Work out the finished part from the listing and answer in its coordinate system (mm). Face numbers are marked on the shaded views. A direction names the side the tool comes from. Give positions to 0.01 mm unless a question says otherwise; leave off trailing zeros. Order: outer loops, then holes, each group sorted by start corner. A loop starts at its lowest first (then second) coordinate and runs counter-clockwise, first axis right, second up. Notation, with made-up numbers: (-21, -32) -> (-1, -32) arc R23 cw to (-1, -23) -> close; hole circle Ø8 at (5.25, -1). An arc over 180 degrees is marked (long way). Answer as CSV lines item,"result". Start each with the question number.
1. A cutting plane is placed at A-A (y = 4.5). Give the vertices of the cut face in (x, z), then the cut area to 3 significant figures.
2. Flat-ended cylindrical pins translate along their axes: pin 1 (15.5 mm diameter, centred on x = -0.5, y = 18.5, fed in from -Z); pin 2 (8 mm diameter, centred on x = 31.5, z = 10, fed in from -Y); pin 3 (3 mm diameter, centred on x = -41, z = 5.5, fed in from -Y); pin 4 (9.5 mm diameter, centred on y = 15.5, z = 14, fed in from +X). Find the tip coordinate at first contact, or state that the pin passes through.
3. A cutting plane is placed at C-C (x = -32.5). Give the vertices of the cut face in (y, z) (1 decimal), then the cut area to 3 significant figures.
4. For the marked faces 5, 6 and 7, determine the directions among +Z, -Z, +X, -X, +Y, -Y from which every point of the face is accessible in a straight line to the end or side of a thin tool.
5. Find the intervals of material crossed by L1, parallel to X at y = 6.5, z = 2.75; L2, parallel to Y at x = 36.5, z = 11.75; L3, parallel to X at y = 4, z = 7.75, in increasing order.
6. For a pull along Y with two mould halves and no side action, classify the marked faces 1, 2, 3 and 4 as released by +Y, released by -Y, zero draft, split by the parting line, or undercut.
7. A cutting plane is placed at B-B (z = 5.25). State how many separate pieces and enclosed holes the cut face has, then the cut area to 3 significant figures.
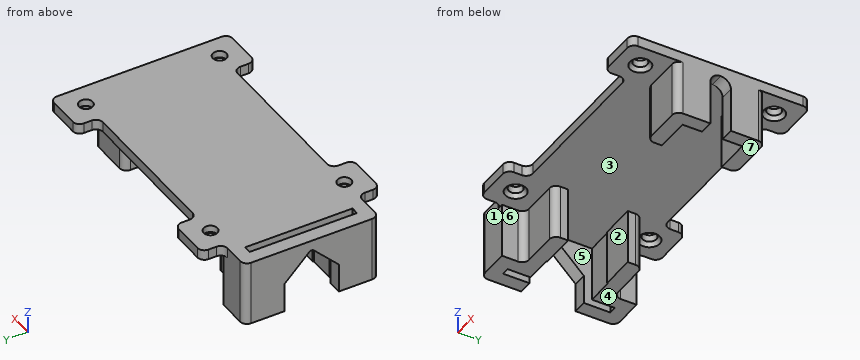
Autodesk Inventor part; units mm, degrees
ref_plane "YZ Plane" through (0, 0, 0) normal (1, 0, 0) x (0, 1, 0)
ref_plane "XZ Plane" through (0, 0, 0) normal (0, 1, 0) x (-1, 0, 0)
ref_plane "XY Plane" through (0, 0, 0) normal (0, 0, 1) x (1, 0, 0)
sketch "Sketch1" plane through (0, 0, 0) normal (0, 0, 1) x (1, 0, 0)
  line L0 (-33.557, 36.1315) -> (-43.657, 36.1315)
  line L1 (-43.657, 36.1315) -> (-43.657, -3.0685)
  line L2 (-43.657, -3.0685) -> (-33.457, -3.0685)
  line L3 (40.043, 3.5815) -> (40.043, 29.4815)
  line L4 (35.943, 25.1065) -> (35.943, 7.9565) construction
  line L5 (35.943, 7.9565) -> (-29.957, 7.9565) construction
  line L6 (35.943, 25.1065) -> (-29.957, 25.1065) construction
  line L7 (-37.557, 25.3815) -> (-29.957, 25.3815) construction
  line L8 (-29.957, 7.6815) -> (-29.957, 25.3815) construction
  line L9 (-37.557, 7.6815) -> (-29.957, 7.6815) construction
  line L10 (-37.557, 1.0315) -> (-37.557, 6.1295) construction
  line L11 (-39.557, 1.0315) -> (-37.557, 1.0315) construction
  line L12 (-39.557, 6.1295) -> (-39.557, 1.0315) construction
  line L13 (-39.557, 13.2232) -> (-39.557, 6.1295) construction
  line L14 (-39.557, 19.8398) -> (-39.557, 13.2232) construction
  line L15 (-39.557, 26.9336) -> (-39.557, 19.8398) construction
  line L16 (-39.557, 32.0315) -> (-39.557, 26.9336) construction
  line L17 (-39.557, 32.0315) -> (-37.557, 32.0315) construction
  line L18 (-37.557, 26.9336) -> (-37.557, 32.0315) construction
  line L19 (-37.557, 19.8398) -> (-37.557, 26.9336) construction
  line L20 (-37.557, 6.1295) -> (-37.557, 13.2232) construction
  line L21 (-33.557, 36.1315) -> (-33.557, 29.4815) construction
  line L22 (-33.557, 29.4815) -> (40.043, 29.4815) construction
  line L23 (35.943, 25.1065) -> (-29.957, 25.1065) construction
  line L24 (-29.957, 25.3815) -> (-29.957, 25.1065) construction
  line L25 (-29.957, 25.3815) -> (-37.557, 25.3815) construction
  line L26 (-37.557, 25.3815) -> (-37.557, 32.0315) construction
  line L27 (-37.557, 32.0315) -> (-39.557, 32.0315) construction
  line L28 (-39.557, 32.0315) -> (-39.557, 1.0315) construction
  line L29 (-39.557, 1.0315) -> (-37.557, 1.0315) construction
  line L30 (-37.557, 1.0315) -> (-37.557, 7.6815) construction
  line L31 (-37.557, 7.6815) -> (-29.957, 7.6815) construction
  line L32 (-29.957, 7.6815) -> (-29.957, 7.9565) construction
  line L33 (-29.957, 7.9565) -> (35.943, 7.9565) construction
  line L34 (35.943, 7.9565) -> (35.943, 25.1065) construction
  line L35 (-29.857, 7.8565) -> (36.043, 7.8565)
  line L36 (36.043, 7.8565) -> (36.043, 25.2065)
  line L37 (36.043, 25.2065) -> (-29.857, 25.2065)
  line L38 (-29.857, 25.2065) -> (-29.857, 25.4815)
  line L39 (-29.857, 25.4815) -> (-37.457, 25.4815)
  line L40 (-37.457, 25.4815) -> (-37.457, 32.1315)
  line L41 (-37.457, 32.1315) -> (-39.657, 32.1315)
  line L42 (-39.657, 32.1315) -> (-39.657, 0.9315)
  line L43 (-39.657, 0.9315) -> (-37.457, 0.9315)
  line L44 (-37.457, 0.9315) -> (-37.457, 7.5815)
  line L45 (-37.457, 7.5815) -> (-29.857, 7.5815)
  line L46 (-29.857, 7.5815) -> (-29.857, 7.8565)
  line L47 (-33.557, 36.1315) -> (-33.557, 29.4815)
  line L48 (-33.557, 29.4815) -> (40.043, 29.4815)
  line L49 (-33.457, -3.0685) -> (-33.457, 3.5815)
  line L50 (-33.457, 3.5815) -> (40.043, 3.5815)
  line L51 (-33.457, 36.1315) -> (-33.557, 36.1315)
  line L52 (-33.457, 36.1315) -> (-33.557, 36.1315)
  point P0 (0, 0)
  dimension "d6" = 0.1
  dimension "d7" = 4
  dimension "d8" = 4
  dimension "d9" = 4
  dimension "d10" = 4
  dimension "d11" = 4
  dimension "d12" = 4
  dimension "d13" = 4
  dimension "d14" = 4
extrude "Extrusion1" add sketch "Sketch1" along normal blind 16
sketch "Sketch2" plane through (0, 0, 16) normal (0, 0, 1) x (1, 0, 0)
  line L0 (-43.657, 36.1315) -> (-43.657, -3.0685)
  line L1 (-43.657, -3.0685) -> (-43.657, 36.1315)
  line L2 (40.043, 36.1315) -> (40.043, -3.0685)
  line L3 (-43.657, -3.0685) -> (-33.457, -3.0685)
  line L4 (40.043, 3.5815) -> (40.043, 29.4815)
  line L5 (40.043, 29.4815) -> (27.043, 29.4815) construction
  line L6 (27.043, 36.1315) -> (27.043, 42.4815)
  line L7 (27.043, 42.4815) -> (40.043, 42.4815)
  line L8 (40.043, 42.4815) -> (40.043, 29.4815)
  line L9 (-33.557, 29.4815) -> (-33.557, 36.1315) construction
  line L10 (-33.557, 29.4815) -> (-20.557, 29.4815) construction
  line L11 (-20.557, 36.1315) -> (-20.557, 42.4815)
  line L12 (-20.557, 42.4815) -> (-33.557, 42.4815)
  line L13 (-33.557, 42.4815) -> (-33.557, 36.1315)
  line L14 (-33.457, 3.5815) -> (40.043, 3.5815) construction
  line L15 (-20.557, 3.5815) -> (-20.457, 3.5815)
  line L16 (-20.457, -3.0685) -> (-20.457, -9.4185)
  line L17 (-20.457, -9.4185) -> (-33.457, -9.4185)
  line L18 (-33.457, -9.4185) -> (-33.457, -3.0685)
  line L19 (40.043, 3.5815) -> (27.043, 3.5815) construction
  line L20 (27.043, -3.0685) -> (27.043, -9.4185)
  line L21 (27.043, -9.4185) -> (40.043, -9.4185)
  line L22 (40.043, -9.4185) -> (40.043, 3.5815)
  line L23 (27.043, -3.0685) -> (-20.457, -3.0685)
  line L24 (-33.457, -3.0685) -> (-43.657, -3.0685)
  line L25 (-43.657, 36.1315) -> (-33.557, 36.1315)
  line L26 (-20.557, 36.1315) -> (27.043, 36.1315)
  point P0 (0, 0)
  point P1 (-38.557, -3.0685)
  point P2 (40.043, 16.5315)
  dimension "d60" = 13
  dimension "d61" = 13
  dimension "d62" = 13
  dimension "d63" = 13
  dimension "d64" = 13
  dimension "d65" = 13
  dimension "d66" = 13
  dimension "d67" = 13
extrude "Extrusion2" add sketch "Sketch2" along normal blind 3
sketch "Sketch3" plane through (40.043, 3.5815, 0) normal (1, 0, 0) x (0, 0, -1)
  line L0 (0, 15.95) -> (-16, 15.95)
  line L1 (-16, 15.95) -> (-16, 9.95)
  line L2 (-16, 9.95) -> (0, 9.95)
  line L3 (0, 9.95) -> (0, 15.95)
  line L4 (0, 0) -> (0, 25.9) construction
  line L5 (0, 25.9) -> (-16, 25.9) construction
  line L6 (0, 0) -> (-16, 0) construction
  line L7 (-16, 21.625) -> (-16, 4.275) construction
  point P0 (0, -3.5815)
  point P1 (0, 12.95)
  dimension "d19" = 6
  dimension "d21" = 0
extrude "Extrusion3" cut sketch "Sketch3" against normal blind 4
fillet "Fillet1" radius 3 2 edges at (38.043, 19.5315, 16) (38.043, 13.5315, 16)
sketch "Sketch4" plane through (-43.657, -3.0685, 0) normal (-1, 0, 0) x (0, 0, 1)
  line L0 (0, 27.5) -> (16, 27.5)
  line L1 (16, 27.5) -> (16, 11.7)
  line L2 (16, 11.7) -> (0, 11.7)
  line L3 (0, 11.7) -> (0, 27.5)
  line L4 (0, 39.2) -> (0, 0) construction
  line L5 (0, 39.2) -> (19, 39.2) construction
  line L6 (0, 0) -> (19, 0) construction
  line L7 (19, 39.2) -> (19, 0) construction
  point P0 (0, 3.0685)
  point P1 (0, 19.6)
  dimension "d25" = 15.8
  dimension "d28" = 11.7
  dimension "d29" = 11.7
  dimension "d30" = 3
extrude "Extrusion4" cut sketch "Sketch4" against normal blind 4
chamfer "Chamfer1" distance 7.5 angle 45 2 edges at (-41.657, 8.6315, 16) (-41.657, 24.4315, 16)
sketch "Sketch5" plane through (0, 0, 16) normal (0, 0, -1) x (-1, 0, 0)
  circle A0 centre (-33.543, 35.9815) radius 2
  circle A1 centre (27.057, 35.9815) radius 2
  circle A2 centre (27.057, -2.9185) radius 2
  circle A3 centre (-33.543, -2.9185) radius 2
  line L0 (-40.043, 29.4815) -> (-40.043, 3.5815)
  line L1 (-40.043, 36.1315) -> (33.557, 36.1315)
  line L2 (-40.043, 29.4815) -> (33.557, 29.4815)
  line L3 (-40.043, -9.4185) -> (-40.043, 3.5815)
  line L4 (33.457, -3.0685) -> (-27.043, -3.0685)
  line L5 (33.457, -3.0685) -> (33.457, 3.5815)
  line L6 (20.557, 42.4815) -> (33.557, 42.4815)
  line L7 (33.457, -9.4185) -> (20.457, -9.4185)
  line L8 (-27.043, -9.4185) -> (-40.043, -9.4185)
  point P0 (0, 0)
  point P1 (-40.043, -3.0685)
  point P2 (27.057, 42.4815)
  point P3 (-33.543, -9.4185)
  dimension "d39" = 4
  dimension "d68" = 6.5
  dimension "d69" = 6.5
extrude "Extrusion5" cut sketch "Sketch5" against normal blind 4
chamfer "Chamfer2" distance 1 angle 45 4 edges at (35.543, 35.9815, 16) (35.543, -2.9185, 16) (-25.057, 35.9815, 16) (-25.057, -2.9185, 16)
chamfer "Chamfer3" distance 0.275 angle 45 2 edges at (-29.857, 25.2065, 8) (-29.857, 7.8565, 8)
sketch "Sketch6" plane through (0, 0, 0) normal (0, 0, -1) x (-1, 0, 0)
  line L0 (37.457, 0.9315) -> (39.657, 0.9315)
  line L1 (39.657, 32.1315) -> (37.457, 32.1315)
  line L2 (37.457, 32.1315) -> (37.457, 0.9315)
  line L3 (37.457, 0.9315) -> (39.657, 0.9315)
  line L4 (39.657, 0.9315) -> (39.657, 32.1315)
  point P0 (0, 0)
extrude "Extrusion6" cut sketch "Sketch6" against normal through all
sketch "Sketch7" plane through (-33.557, 29.4815, 0) normal (0, 1, 0) x (1, 0, 0)
  line L0 (3.7, 0) -> (3.7, -16) construction
  line L1 (3.975, -16) -> (3.975, 0) construction
  line L2 (69.6, 0) -> (69.6, -16) construction
  line L3 (13.975, 0) -> (59.6, 0)
  line L4 (59.6, 0) -> (59.6, -16)
  line L5 (59.6, -16) -> (13.975, -16)
  line L6 (13.975, -16) -> (13.975, 0)
  line L7 (73.6, -16) -> (0, -16) construction
  point P0 (33.557, 0)
  point P1 (36.7875, -16)
  point P2 (36.8, -16)
  dimension "d56" = 10
  dimension "d57" = 10
extrude "Extrusion7" cut sketch "Sketch7" against normal through all
fillet "Fillet2" radius 2 24 edges at (-33.557, 42.4815, 17.5) (-20.557, 42.4815, 17.5) (27.043, 42.4815, 17.5) (40.043, 42.4815, 17.5) (27.043, -9.4185, 17.5) (40.043, -9.4185, 17.5) (-20.457, -9.4185, 17.5) (-33.457, -9.4185, 17.5) (-43.657, -3.0685, 9.5) (-43.657, 36.1315, 9.5) (-19.582, 29.4815, 8) (-19.582, 3.5815, 8) (40.043, 29.4815, 8) (40.043, 3.5815, 8) (26.043, 3.5815, 8) (26.043, 29.4815, 8) (27.043, 36.1315, 17.5) (-20.557, 36.1315, 17.5) (-33.557, 36.1315, 17.5) (-33.557, 29.4815, 8) (-33.457, 3.5815, 8) (-20.457, -3.0685, 17.5) (27.043, -3.0685, 17.5) (-33.457, -3.0685, 17.5)
equation "\"d28\" = d29"
equation "\"d69\" = d68"
properties part number "SyringeCasing"
Answer sheet:
1,outline,"(-43.66, 0) -> (-39.66, 0) -> (-39.66, 19) -> (-43.66, 19) -> close; (-37.46, 0) -> (-19.9, 0) -> (-19.9, 16) -> (26.36, 16) -> (26.36, 0) -> (39.73, 0) -> (39.73, 16) -> (40.04, 16) -> (40.04, 19) -> (-37.46, 19) -> close"
1,area,"803 mm^2"
2,pin 1,"stops at z = 16"
2,pin 2,"stops at y = 3.58"
2,pin 3,"stops at y = -3.07"
2,pin 4,"stops at x = 40.04"
3,outline,"(-9.1, 16) -> (3.3, 16) -> (3.3, 0) -> (7.6, 0) -> (7.6, 16) -> (25.5, 16) -> (25.5, 0) -> (29.7, 0) -> (29.7, 16) -> (42.2, 16) -> (42.2, 19) -> (-9.1, 19) -> close"
3,area,"291 mm^2"
4,face 5,"+Z, -Z"
4,face 6,"-Z, +X, -Y"
4,face 7,"-Z, +X, -X, +Y, -Y"
5,L1,"x = -43.66 to -39.66, -37.46 to -19.58, 26.04 to 40.04"
5,L2,"y = 3.58 to 13.53, 19.53 to 29.48"
5,L3,"x = -43.66 to -39.66, -37.46 to -20.36, 26.82 to 39.27"
6,face 1,"released by -Y"
6,face 2,"undercut"
6,face 3,"undercut"
6,face 4,"zero draft"
7,separate pieces,"4"
7,enclosed holes,"0"
7,area,"472 mm^2"
